from build123d import *

# Parameters (mm, degrees)
SKETCH1_W = 3.5
SKETCH1_H = 11


with BuildPart() as part:
    # Sketch1 → Revolve1 (revolve)
    with BuildSketch(Plane.XY, mode=Mode.PRIVATE) as revolve1_sk:
        with BuildLine():
            Line((9.085974676, 39), (3.5, 39))
            Line((3.5, 39), (3.5, 28))
            Line((3.5, 28), (0, 28))
            Line((0, 28), (0, -39))
            ThreePointArc((0, -39), (7.778174593, -35.778174593), (11, -28))
            Line((11, -28), (11, 36.706189904))
            add(Edge.make_bspline(
                [(9.085974676, 39), (9.952667981, 38.554296202), (10.670284632, 37.900307222), (11, 36.706189904)],
                knots=[0.726528094, 0.726528094, 0.726528094, 0.726528094, 1, 1, 1, 1], degree=3))
        make_face()
        with BuildLine():
            Line((3.5, 44.089340843), (3.5, 39))
            Line((3.5, 39), (9.085974676, 39))
            add(Edge.make_bspline(
                [(3.5, 44.089340843), (3.569121253, 39.909476787), (6.831780935, 40.159236729), (9.085974676, 39)],
                knots=[0.015251506, 0.015251506, 0.015251506, 0.015251506, 0.726528094, 0.726528094, 0.726528094, 0.726528094], degree=3))
        make_face()
        with Locations((1.75, 33.5)):
            Rectangle(SKETCH1_W, SKETCH1_H)
        with BuildLine():
            Line((0, 50), (0, 39))
            Line((0, 39), (3.5, 39))
            Line((3.5, 39), (3.5, 44.089340843))
            add(Edge.make_bspline(
                [(3.5, 44.364387792), (3.498504063, 44.270630457), (3.498517872, 44.178967328), (3.5, 44.089340843)],
                knots=[0, 0, 0, 0, 0.015251506, 0.015251506, 0.015251506, 0.015251506], degree=3))
            Line((3.5, 44.364387792), (3.5, 50))
            Line((3.5, 50), (0, 50))
        make_face()
    revolve(revolve1_sk.sketch.rotate(Axis((0, 28, 0), (0, -1, 0)), 180), axis=Axis((0, 28, 0), (0, -1, 0)))


solid = part.part
Can you work these out from the model? Positions are in its coordinate system, mm. A direction names the side the tool comes from. Coordinates: 2 decimals unless noted, no trailing zeros. Order: outer loops, then holes, each group sorted by start corner. A loop starts at its lowest first (then second) coordinate and runs counter-clockwise, first axis right, second up. Notation, with made-up numbers: (-9, 53) - (26, 53) arc R34 cw to (26, 85) - close; hole circle Ø4 at (2.5, 37.25). An arc over 180 degrees is marked (long way). Answer as a JSON object with one key per item and string values. Group by question number.
Q1. I need wall thicknesses on line 1 (Z direction, x = 0.5, y = -17.5); line 2 (X direction, y = -14.5, z = -1.25). Which ranges of each line are inside material? Lowest first, please. Write a range as from..to.
Q2. Imagine slicing it at A-A (y = -10). Please give me the cut outline in (x, z).
Q3. Imagine slicing it at B-B (y = -31). Please give me the cut outline in (x, z), and give its area (3 significant figures).
Q4. On a 3-axis mill with a long thin cutter (end or side, diameter ignored), from which of +Z, -Z, +X, -X, +Y, -Y can I reach the whole of each face in a straight line? I mean faces 1 (the face through (2.38, 4.81, 10.74)), 2 (the face through (-3.233, 47.222, 1.341)). Say none if no direction works.
Q5. Will these pins go through, and if not, where does the flat tip stop? P1, Ø1.5, axis at y = 11, z = 2, coming from the -X side; P2, Ø3, axis at y = 7, z = -7, coming from the +X side; P3, Ø5, axis at x = 0.5, z = 4, coming from the -Y side.
Determined:
{
 "1": {"line 1": "z = -10.99..10.99", "line 2": "x = -10.93..10.93"},
 "2": {"outline": "circle Ø22 at (0, 0)"},
 "3": {"outline": "circle Ø21.17 at (0, 0)", "area": "352 mm2"},
 "4": {"face 1": "+Y, -Y", "face 2": "+Y"},
 "5": {"P1": "stops at x = -10.93", "P2": "stops at x = 9.53", "P3": "stops at y = -38.89"}
}
